Can you work these out from the model? Positions are in its coordinate system, mm. A direction names the side the tool comes from. Give positions to 0.01 mm unless a question says otherwise; leave off trailing zeros. Order: outer loops, then holes, each group sorted by start corner. A loop starts at its lowest first (then second) coordinate and runs counter-clockwise, first axis right, second up. Notation, with made-up numbers: (-13.75, -37.5) -> (40.25, -37.5) arc R26 cw to (40.25, -17.5) -> close; hole circle Ø8 at (75, 49.5). An arc over 180 degrees is marked (long way). Answer as a JSON object with one key per item and string values.
```python
from build123d import *

# Parameters (mm, degrees)
SKETCH1_W           = 225
SKETCH1_H           = 225
SKETCH1_W_2         = 210
SKETCH1_H_2         = 210
BOSS_EXTRUDE1_DEPTH = 15
SKETCH2_R           = 3.9
CUT_EXTRUDE1_DEPTH  = 253.004464246
FILLET1_R           = 10
FILLET2_R           = 17.5


with BuildPart() as part:
    # Sketch1 → Boss-Extrude1 (new body)
    with BuildSketch(Plane(origin=(0, 0, 0), x_dir=(0, 1, 0), z_dir=(0, 0, 1))):
        Rectangle(SKETCH1_W, SKETCH1_H)
        Rectangle(SKETCH1_W_2, SKETCH1_H_2, mode=Mode.SUBTRACT)
    extrude(amount=BOSS_EXTRUDE1_DEPTH)

    # Sketch2 → Cut-Extrude1 (cut, through all)
    with BuildSketch(Plane.YZ.offset(112.5)):
        with Locations(Location((-7.8, 7.5, 0), (0, 0, 270))):
            Circle(SKETCH2_R)
        with Locations(Location((7.8, 7.5, 0), (0, 0, 90))):
            Circle(SKETCH2_R)
    extrude(amount=-CUT_EXTRUDE1_DEPTH, mode=Mode.SUBTRACT)

    # Fillet1
    fillet1_edges = [part.edges().sort_by_distance(p)[0] for p in [
        (105, 105, 7.5),
        (-105, 105, 7.5),
        (-105, -105, 7.5),
        (105, -105, 7.5),
    ]]
    fillet(fillet1_edges, radius=FILLET1_R)

    # Fillet2
    fillet2_edges = [part.edges().sort_by_distance(p)[0] for p in [
        (112.5, 112.5, 7.5),
        (112.5, -112.5, 7.5),
        (-112.5, -112.5, 7.5),
        (-112.5, 112.5, 7.5),
    ]]
    fillet(fillet2_edges, radius=FILLET2_R)


solid = part.part
```
1. If we section it at A-A on x = 30: Please give me the cut outline in (y, z), then the cut area to 3 significant figures.
Worked answers:
{"outline": "(-112.5, 0) -> (-105, 0) -> (-105, 15) -> (-112.5, 15) -> close; (105, 0) -> (112.5, 0) -> (112.5, 15) -> (105, 15) -> close", "area": "225 mm²"}
2. If we mould it in two halves opening along X, with no side actions, what happens to faces 1 (the face through (-105, -1, 7)), 2 (the face through (-112.5, -1, 7)), 3 (the face through (1, 112.5, 7))? For each: +X half, -X half, draft (parallel to the pull), parting line (faces both ways), or undercut.
Worked answers:
{"face 1": "undercut", "face 2": "-X half", "face 3": "draft"}
3. If we section it at B-B on z = 7.5: Count the separate pieces of the cut face and the enclosed holes in it, then the cut area to 3 significant figures.
Worked answers:
{"separate pieces": "4", "enclosed holes": "0", "area": "6,110 mm²"}
4. If we section it at C-C on y = -7.8: Please give me the cut outline in (x, z), then the cut area to 3 significant figures.
Worked answers:
{"outline": "(-112.5, 0) -> (-105, 0) -> (-105, 3.6) -> (-112.5, 3.6) -> close; (-112.5, 11.4) -> (-105, 11.4) -> (-105, 15) -> (-112.5, 15) -> close; (105, 0) -> (112.5, 0) -> (112.5, 3.6) -> (105, 3.6) -> close; (105, 11.4) -> (112.5, 11.4) -> (112.5, 15) -> (105, 15) -> close", "area": "108 mm²"}
5. Please list where these lines run through material, in increasing order: L1, parallel to Y at x = -107.25, z = 7.5; L2, parallel to Y at x = -17, z = 12.25.
Worked answers:
{"L1": "-107.5 to -11.7, -3.9 to 3.9, 11.7 to 107.5", "L2": "-112.5 to -105, 105 to 112.5"}
6. For faces 4 (the face through (112.5, -1, 7)), 5 (the face through (102.15, -101.99, 7.6)), which set-ups out of +Z, -Z, +X, -X, +Y, -Y let a thin tool reach every point of the face, with its end or its side?
Worked answers:
{"face 4": "+Z, -Z, +X, +Y, -Y", "face 5": "+Z, -Z"}
